Model file for the job. Use its own axes, mm. Face numbers are marked on the shaded views. Give positions to 0.01 mm unless a question says otherwise; leave off trailing zeros. Write each loop counter-clockwise with the first axis right and the second up, starting at its lowest first coordinate (ties: lowest second). Pieces come first, ordered by that corner, then holes.
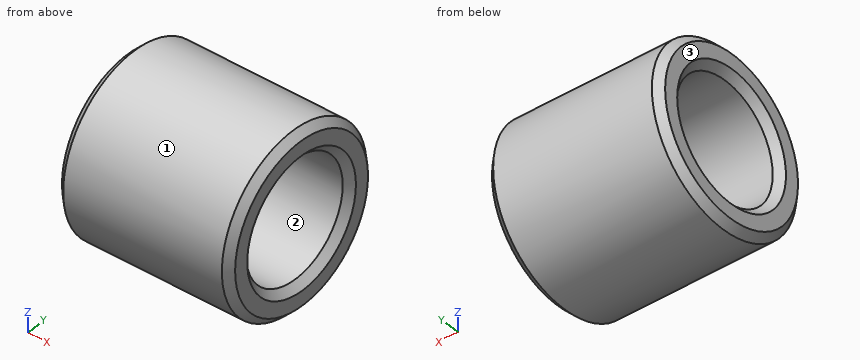
```python
from build123d import *

# Parameters (mm, degrees)
F0_R     = 6
F0_R_2   = 4
F1_DEPTH = 12
F2_SIZE  = 0.5


with BuildPart() as f1:
    # F0 (on Right) → F1 (new body)
    with BuildSketch(Plane.YZ):
        Circle(F0_R)
        Circle(F0_R_2, mode=Mode.SUBTRACT)
    extrude(amount=F1_DEPTH)

    # F2
    f2_edges = [f1.edges().sort_by_distance(p)[0] for p in [
        (12, -6, 0),
        (12, -4, 0),
        (0, -6, 0),
        (0, -4, 0),
    ]]
    chamfer(f2_edges, length=F2_SIZE)


solid = f1.part
```
1. Pin check, flat tips, straight feed: P1, Ø4, axis at x = 2, y = 3, coming from the -Z side; P2, Ø6, axis at x = 2.5, y = 4, coming from the +Z side; P3, Ø5, axis at x = 9.5, y = -3, coming from the +Z side; P4, Ø3, axis at y = 4, z = 1, coming from the -X side. Stop position of each tip, or through.
Calculated:
P1: stops at z = -5.92
P2: stops at z = 5.92
P3: stops at z = 5.98
P4: stops at x = 0
2. Probe probe 1 along Y at (x, z) = (7.75, 1); probe 2 along Z at (x, y) = (6, 1.25); probe 3 along Z at (x, y) = (4, 0). List the from-to ranges inside material, lowest first.
Calculated:
probe 1: y = -5.92 to -3.87, 3.87 to 5.92
probe 2: z = -5.87 to -3.8, 3.8 to 5.87
probe 3: z = -6 to -4, 4 to 6
3. Slice it at C-C, the plane x = 6.25. Write the cut outline in (y, z), and give its area (3 significant figures).
Calculated:
outline: circle Ø12 at (0, 0); hole circle Ø8 at (0, 0)
area: 62.8 mm2
4. Slice it at A-A, the plane z = 0. Write the cut outline in (x, y).
Calculated:
outline: (0, -5.5) - (0.5, -6) - (11.5, -6) - (12, -5.5) - (12, -4.5) - (11.5, -4) - (0.5, -4) - (0, -4.5) - close; (0, 4.5) - (0.5, 4) - (11.5, 4) - (12, 4.5) - (12, 5.5) - (11.5, 6) - (0.5, 6) - (0, 5.5) - close
5. Pull direction Z, two halves, no side cores. Call the marked faces 1, 2 and 3: +Z half, -Z half, draft (parallel to the pull), parting line (faces both ways), or undercut.
Calculated:
face 1: parting line
face 2: undercut
face 3: draft
